```python
from build123d import *

# Parameters (mm, degrees)
F1_DEPTH = 15
F3_DEPTH = 3
F4_R     = 3.4
F5_DEPTH = 18.001


with BuildPart() as f1:
    # F0 (on Top) → F1 (new body)
    with BuildSketch(Plane.XY):
        with BuildLine():
            Line((12.6, 0), (12.6, 22.4))
            ThreePointArc((12.6, 22.4), (11.135534, 25.935534), (7.6, 27.4))
            Line((7.6, 27.4), (0, 27.4))
            Line((0, 27.4), (-7.6, 27.4))
            ThreePointArc((-7.6, 27.4), (-11.135534, 25.935534), (-12.6, 22.4))
            Line((-12.6, 22.4), (-12.6, 0))
            Line((-12.6, 0), (-12.6, -11.6))
            Line((-12.6, -11.6), (0, -11.6))
            Line((0, -11.6), (12.6, -11.6))
            Line((12.6, -11.6), (12.6, 0))
        make_face()
        Polygon((-7.6, 6.6), (0, 6.6), (7.6, 6.6), (7.6, 0), (7.6, -6.6), (0, -6.6), (-7.6, -6.6), (-7.6, 0), align=None, mode=Mode.SUBTRACT)
    extrude(amount=F1_DEPTH)

    # F2 (on face) → F3 (join)
    with BuildSketch(Plane.XY.offset(15)):
        with BuildLine():
            Line((-12.6, 22.4), (-12.6, -11.6))
            Line((-12.6, -11.6), (0, -11.6))
            Line((0, -11.6), (12.6, -11.6))
            Line((12.6, -11.6), (12.6, 22.4))
            ThreePointArc((12.6, 22.4), (11.135534, 25.935534), (7.6, 27.4))
            Line((7.6, 27.4), (0, 27.4))
            Line((0, 27.4), (-7.6, 27.4))
            ThreePointArc((-7.6, 27.4), (-11.135534, 25.935534), (-12.6, 22.4))
        make_face()
    extrude(amount=F3_DEPTH)

    # F4 (on face) → F5 (cut, through all)
    with BuildSketch(Plane.XY.offset(18)):
        with Locations((0, 22.4)):
            Circle(F4_R)
    extrude(amount=-F5_DEPTH, mode=Mode.SUBTRACT)


solid = f1.part
```
Geometry: final body of the model. Coordinates: model frame, mm. A direction names the side the tool comes from. Round coordinates to 2 decimals unless told otherwise and drop trailing zeros. Write each loop counter-clockwise with the first axis right and the second up, starting at its lowest first coordinate (ties: lowest second). Pieces come first, ordered by that corner, then holes. Notation, with made-up numbers: M 73.5,42.25 L 92.5,42.25 A26 ccw 92.5,57.25 Z; hole C -29,-40 d7. An arc over 180 degrees is marked long. Answer in a Markdown table with one row per item. Add a question column.
(1) Cut plane B-B, the plane x = 3. Return the cut outline in (y, z).
(2) Cut plane A-A, the plane y = -4.5. Return the cut outline in (x, z).
(3) Contact query for flat-ended pins moving along their axis: pin 1 (10.5 mm diameter, centred on x = 3.5, y = 2.5, fed in from -Z); pin 2 (5.5 mm diameter, centred on x = 0, y = 22.4, fed in from -Z). Output: stop coordinate, or through.
(4) Reachability of faces 1 (the face through (0, 0, 15)), 2 (the face through (11.17, 25.9, 8.87)) from +Z, -Z, +X, -X, +Y, -Y: full face, straight path, thin tool, end or side. Return the list, or none.
(5) Ray query, L1, parallel to Y at x = 0, z = 5.75; L2, parallel to X at y = 6, z = 6.75; L3, parallel to Y at x = 6, z = 8.75. Return the intervals inside material, ascending.
(6) Draft query along Y for faces 3 (the face through (-7.6, 0, 7)), 4 (the face through (-12.6, 6, 9)), 5 (the face through (-11.1, 25.97, 8.87)). Return one class per face: pulls with the +Y half, pulls with the -Y half, needs draft (parallel to the pull), parting line crosses it, or undercut.
(7) Cut plane D-D, the plane z = 16.5. Return the cut outline in (x, y).
(8) Cut plane C-C, the plane z = 12.5. Return the cut outline in (x, y), then the cut area to 3 significant figures.
Established:
| question | item | result |
|---|---|---|
| 1 | outline | M -11.6,0 L -6.6,0 L -6.6,15 L 6.6,15 L 6.6,0 L 20.8,0 L 20.8,18 L -11.6,18 Z; M 24,0 L 27.4,0 L 27.4,18 L 24,18 Z |
| 2 | outline | M -12.6,0 L -7.6,0 L -7.6,15 L 7.6,15 L 7.6,0 L 12.6,0 L 12.6,18 L -12.6,18 Z |
| 3 | pin 1 | z = 0 |
| 3 | pin 2 | through |
| 4 | face 1 | -Z |
| 4 | face 2 | +Z, -Z, +X, +Y |
| 5 | L1 | -11.6 to -6.6, 6.6 to 19, 25.8 to 27.4 |
| 5 | L2 | -12.6 to -7.6, 7.6 to 12.6 |
| 5 | L3 | -11.6 to -6.6, 6.6 to 27.4 |
| 6 | face 3 | undercut |
| 6 | face 4 | needs draft |
| 6 | face 5 | pulls with the +Y half |
| 7 | outline | M -12.6,-11.6 L 12.6,-11.6 L 12.6,22.4 A5 ccw 7.6,27.4 L -7.6,27.4 A5 ccw -12.6,22.4 Z; hole C 0,22.4 d6.8 |
| 8 | outline | M -12.6,-11.6 L 12.6,-11.6 L 12.6,22.4 A5 ccw 7.6,27.4 L -7.6,27.4 A5 ccw -12.6,22.4 Z; hole M -7.6,-6.6 L 7.6,-6.6 L 7.6,6.6 L -7.6,6.6 Z; hole C 0,22.4 d6.8 |
| 8 | area | 735 mm² |
